```python
from build123d import *

# Parameters (mm, degrees)
F0_W          = 4.2
F0_H          = 1.6
F1_DEPTH      = 5.85
F1_DEPTH_BACK = 5.85
F3_DEPTH      = 3.7
F4_R          = 1.9
F5_DEPTH      = 3.6
F6_R          = 1.05
F7_DEPTH      = 10
F9_DEPTH      = 25
F9_DEPTH_BACK = 25
F10_R         = 0.5
F11_R         = 0.5
F12_DEPTH     = 5


with BuildPart() as f1:
    # F0 (on Right) → F1 (new body, two sides)
    with BuildSketch(Plane.YZ) as f1_sk:
        with Locations((-13.95, 15.85)):
            Rectangle(F0_W, F0_H)
        with Locations((13.95, 15.85)):
            Rectangle(F0_W, F0_H)
        Polygon((11.85, 20.6), (-11.85, 20.6), (-11.85, 16.65), (-11.85, 15.05), (-11.85, 0), (11.85, 0), (11.85, 15.05), (11.85, 16.65), align=None)
    extrude(amount=F1_DEPTH)
    extrude(f1_sk.sketch, amount=-F1_DEPTH_BACK)

    # F2 (on face) → F3 (join)
    with BuildSketch(Plane.XY.offset(20.6)):
        with BuildLine():
            ThreePointArc((3.1937438845, 1.65), (4.9621046822, 3.6543272311), (5.6, 6.25))
            ThreePointArc((5.6, 6.25), (-2.5956727689, 11.2121046822), (-3.1937438845, 1.65))
            ThreePointArc((-3.1937438845, 1.65), (-3.064580666, 1.5629598528), (-2.9330467827, 1.4795454545))
            ThreePointArc((-2.9330467827, 1.4795454545), (0, 3.4), (2.9330467827, 1.4795454545))
            ThreePointArc((2.9330467827, 1.4795454545), (3.064580666, 1.5629598528), (3.1937438845, 1.65))
        make_face()
        with BuildLine():
            ThreePointArc((-2.9330467827, 1.4795454545), (-3.064580666, 1.5629598528), (-3.1937438845, 1.65))
            Line((-3.1937438845, 1.65), (-3.1937438845, 0.4))
            ThreePointArc((-3.1937438845, 0.4), (-3.1105860488, 0.9511687112), (-2.9330467827, 1.4795454545))
        make_face()
        with BuildLine():
            Line((3.1937438845, 0.4), (3.1937438845, 1.65))
            ThreePointArc((3.1937438845, 1.65), (3.064580666, 1.5629598528), (2.9330467827, 1.4795454545))
            ThreePointArc((2.9330467827, 1.4795454545), (3.1105860488, 0.9511687112), (3.1937438845, 0.4))
        make_face()
        with BuildLine():
            ThreePointArc((2.9330467827, 1.4795454545), (0, 0.65), (-2.9330467827, 1.4795454545))
            ThreePointArc((-2.9330467827, 1.4795454545), (-3.1105860488, 0.9511687112), (-3.1937438845, 0.4))
            Line((-3.1937438845, 0.4), (-3.1937438845, 0))
            ThreePointArc((-3.1937438845, 0), (0, -3), (3.1937438845, 0))
            Line((3.1937438845, 0), (3.1937438845, 0.4))
            ThreePointArc((3.1937438845, 0.4), (3.1105860488, 0.9511687112), (2.9330467827, 1.4795454545))
        make_face()
        with BuildLine():
            Line((-3.1937438845, 0), (-3.1937438845, 0.4))
            ThreePointArc((-3.1937438845, 0.4), (-3.2, 0.2), (-3.1937438845, 0))
        make_face()
        with BuildLine():
            ThreePointArc((3.2, 0.2), (3.1984355887, 0.3000489118), (3.1937438845, 0.4))
            Line((3.1937438845, 0.4), (3.1937438845, 0))
            ThreePointArc((3.1937438845, 0), (3.1984355887, 0.0999510882), (3.2, 0.2))
        make_face()
        with BuildLine():
            ThreePointArc((-2.9330467827, 1.4795454545), (0, 0.65), (2.9330467827, 1.4795454545))
            ThreePointArc((2.9330467827, 1.4795454545), (0, 3.4), (-2.9330467827, 1.4795454545))
        make_face()
    extrude(amount=F3_DEPTH)

    # F4 (on face) → F5 (join)
    with BuildSketch(Plane.XY.offset(24.3)):
        with Locations((0, 6.25)):
            Circle(F4_R)
    extrude(amount=F5_DEPTH)

    # F6 (on face) → F7 (cut)
    with BuildSketch(Plane.XY.offset(16.65)):
        with Locations((0, 13.75)):
            Circle(F6_R)
        with Locations((0, -13.75)):
            Circle(F6_R)
    extrude(amount=-F7_DEPTH, mode=Mode.SUBTRACT)

    # F8 (on Right) → F9 (cut, two sides)
    with BuildSketch(Plane.YZ) as f9_sk:
        Polygon((11.85, 3), (6.85, 0), (11.85, 0), align=None)
    extrude(amount=-F9_DEPTH, mode=Mode.SUBTRACT)
    extrude(f9_sk.sketch, amount=F9_DEPTH_BACK, mode=Mode.SUBTRACT)

    # F10
    f10_edges = [f1.edges().sort_by_distance(p)[0] for p in [
        (5.85, -11.85, 18.625),
        (-5.85, -11.85, 18.625),
        (-5.85, -11.85, 7.525),
        (5.85, -11.85, 7.525),
        (5.85, 11.85, 18.625),
        (-5.85, 11.85, 18.625),
        (-5.85, 11.85, 9.025),
        (5.85, 11.85, 9.025),
        (5.85, 16.05, 15.85),
        (-5.85, 16.05, 15.85),
        (5.85, -16.05, 15.85),
        (-5.85, -16.05, 15.85),
    ]]
    fillet(f10_edges, radius=F10_R)

    # F11 (on face) → F12 (join)
    with BuildSketch(Plane(origin=(0, 11.85, 0), x_dir=(-1, 0, 0), z_dir=(0, 1, 0))):
        with Locations((0, 3.6)):
            Circle(F11_R)
        with Locations((1.025, 3.6)):
            Circle(F11_R)
        with Locations((-1.025, 3.6)):
            Circle(F11_R)
    extrude(amount=F12_DEPTH)


solid = f1.part
```
Model file for the job. Use its own axes, mm. A direction names the side the tool comes from. Coordinates: 2 decimals unless noted, no trailing zeros. Order: outer loops, then holes, each group sorted by start corner. A loop starts at its lowest first (then second) coordinate and runs counter-clockwise, first axis right, second up. Notation, with made-up numbers: (-30, 14.5) - (24, 14.5) arc R20 ccw to (24, 29.5) - close; hole circle Ø6 at (56, 63). An arc over 180 degrees is marked (long way). Return JSON: item names as keys, results as strings. Group by question number.
1) Mould opens along Z. For faces 4 (the flat face through (0, -11.85, 19)), 5 (the cylindrical face through (-0.3, 14.3, 4)), 6 (the flat face through (0, -3, 0)), 7 (the flat face through (0, 6, 27.9)) say: released by +Z, released by -Z, zero draft, split by the parting line, or undercut.
2) Probe line 1 (Y direction, x = 0, z = 15.6); line 2 (Z direction, x = -3.75, y = 5); line 3 (Y direction, x = 0.5, z = 20). List the from-to ranges inside material, lowest first. Write a range as from..to.
3) Saw through at D-D, the plane x = -2.75. Write the cut outline in (y, z), plus the area to 3 significant figures.
4) Tool access for faces 1 (the cylindrical face through (-0.247, 8.134, 26.075)), 2 (the flat face through (0, -11.85, 8)), 3 (the flat face through (0, 16.05, 16)): list every direction of +Z, -Z, +X, -X, +Y, -Y with a clear straight run to the whole face (end or side of a thin tool).
5) Saw through at A-A, the plane y = -13.75. Write the cut outline in (x, z), plus the area to 3 significant figures.
6) Saw through at C-C, the plane y = 13.75. Write the cut outline in (x, z) (3 decimals).
7) Saw through at B-B, the plane z = 3.6. Write the cut outline in (x, y) (3 decimals).
8) Flat gauge pins, fed straight in: P1, Ø0.6, axis at y = 1.5, z = 22, coming from the +X side; P2, Ø2, axis at x = -2, z = 4, coming from the -Y side; P3, Ø1.4, axis at x = 0.5, y = -14.5, coming from the -Z side; P4, Ø1.3, axis at x = 0, y = -13.75, coming from the -Z side. Where does each tip first touch, or does it go through?
Values found:
{
 "1": {"face 4": "zero draft", "face 5": "undercut", "face 6": "released by -Z", "face 7": "released by +Z"},
 "2": {"line 1": "y = -16.05..-14.8, -12.7..12.7, 14.8..16.05", "line 2": "z = 0..24.3", "line 3": "y = -11.85..11.85"},
 "3": {"outline": "(-16.05, 15.05) - (-11.85, 15.05) - (-11.85, 0) - (6.85, 0) - (11.85, 3) - (11.85, 15.05) - (16.05, 15.05) - (16.05, 16.65) - (11.85, 16.65) - (11.85, 20.6) - (11.13, 20.6) - (11.13, 24.3) - (-1.44, 24.3) - (-1.44, 20.6) - (-11.85, 20.6) - (-11.85, 16.65) - (-16.05, 16.65) - close", "area": "541 mm²"},
 "4": {"face 1": "+Z", "face 2": "-Z, +X, -X, -Y", "face 3": "+Z, +X, -X, +Y"},
 "5": {"outline": "(-5.85, 15.05) - (-1.05, 15.05) - (-1.05, 16.65) - (-5.85, 16.65) - close; (1.05, 15.05) - (5.85, 15.05) - (5.85, 16.65) - (1.05, 16.65) - close", "area": "15.4 mm²"},
 "6": {"outline": "(-5.85, 15.05) - (-1.05, 15.05) - (-1.05, 16.65) - (-5.85, 16.65) - close; circle Ø1 at (-1.025, 3.6); circle Ø1 at (0, 3.6); circle Ø1 at (1.025, 3.6); (1.05, 15.05) - (5.85, 15.05) - (5.85, 16.65) - (1.05, 16.65) - close"},
 "7": {"outline": "(-5.85, -11.35) arc R0.5 ccw to (-5.35, -11.85) - (5.35, -11.85) arc R0.5 ccw to (5.85, -11.35) - (5.85, 11.35) arc R0.5 ccw to (5.35, 11.85) - (1.525, 11.85) - (1.525, 16.85) - (0.525, 16.85) - (0.525, 11.85) - (0.5, 11.85) - (0.5, 16.85) - (-0.5, 16.85) - (-0.5, 11.85) - (-0.525, 11.85) - (-0.525, 16.85) - (-1.525, 16.85) - (-1.525, 11.85) - (-5.35, 11.85) arc R0.5 ccw to (-5.85, 11.35) - close"},
 "8": {"P1": "stops at x = 3.4", "P2": "stops at y = -11.85", "P3": "stops at z = 15.05", "P4": "passes through"}
}
